Source: CAD feature listing. Evaluate the final solid. Frame: model axes, mm. Round coordinates to 2 decimals unless told otherwise and drop trailing zeros. Order: outer loops, then holes, each group sorted by start corner. A loop starts at its lowest first (then second) coordinate and runs counter-clockwise, first axis right, second up. Notation, with made-up numbers: M 38.5,58.25 L 83.5,58.25 A32 cw 83.5,84.25 Z; hole C 31.5,-5.5 d1. An arc over 180 degrees is marked long. Answer as CSV lines item,"result". Start each with the question number.
Item 1: Line query: line 1 (X direction, y = 1, z = 0); line 2 (X direction, y = 0.25, z = -11.43); line 3 (X direction, y = 4.75, z = 1). Output: solid intervals per line, ascending. Write a range as [from, to].
Item 2: Pull-direction query (Z, two-part tool) for faces 1 (the face through (-47, 5.08, 0)), 2 (the face through (-45.05, 0.07, 12.29)), 3 (the face through (-122.64, 0.03, -1.07)), 4 (the face through (-88.502, 0.763, 2.423)); classes: +Z half, -Z half, draft (parallel to the pull), parting line (faces both ways), or undercut.
Item 3: Section query C-C on y = -3.5. Return the cut outline in (x, z).
Item 4: Section query D-D on x = -94. Return the cut outline in (y, z), plus the area to 3 significant figures.
Item 5: Section query A-A on y = 0. Return the cut outline in (x, z).
Item 6: Section query B-B on z = 0. Return the cut outline in (x, y).
Item 7: First-contact query: P1, Ø3.5, axis at x = -47.13, z = -11.43, coming from the +Y side; P2, Ø3, axis at x = -55, z = 2, coming from the -Y side; P3, Ø1, axis at x = -116, y = -2, coming from the -Z side; P4, Ø6, axis at y = -3.5, z = -11.5, coming from the -X side. Flat tips, straight axial feed; report the tip coordinate or a pass-through.
from build123d import *

# Parameters (mm, degrees)
BOSS_EXTRUDE1_DEPTH = 5.08
CUT_EXTRUDE1_REACH  = 12.16
SKETCH4_R           = 2.2479
SKETCH5_R           = 2.54
BOSS_EXTRUDE2_DEPTH = 76.2
CUT_EXTRUDE5_REACH  = 9.62
SKETCH6_R           = 1.27


with BuildPart() as part:
    # Sketch2 → Boss-Extrude1 (new body, symmetric)
    with BuildSketch(Plane(origin=(0, 0, 0), x_dir=(1, 0, 0), z_dir=(0, 1, 0))):
        with BuildLine():
            Line((-50.935337995, 2.421627074), (-50.935337995, -2.138056527))
            Line((-50.935337995, -2.138056527), (-50.935337995, -11.43))
            ThreePointArc((-50.935337995, -11.43), (-47.125337995, -15.24), (-43.315337995, -11.43))
            Line((-43.315337995, -11.43), (-43.315337995, 11.43))
            ThreePointArc((-43.315337995, 11.43), (-47.125337995, 15.24), (-50.935337995, 11.43))
            Line((-50.935337995, 11.43), (-50.935337995, 2.421627074))
        make_face()
    extrude(amount=BOSS_EXTRUDE1_DEPTH, both=True)

    # Sketch4 → Cut-Extrude1 (cut, up to next)
    with BuildSketch(Plane(origin=(0, 5.08, 0), x_dir=(1, 0, 0), z_dir=(0, 1, 0)), mode=Mode.PRIVATE) as cut_extrude1_sk1:
        with Locations((-47.125337995, 11.43)):
            Circle(SKETCH4_R)
    cut_extrude1_tool1 = extrude(cut_extrude1_sk1.sketch, amount=-CUT_EXTRUDE1_REACH, mode=Mode.PRIVATE) & part.part
    add(cut_extrude1_tool1.solids().sort_by_distance((-47.125338, 5.08, -11.43))[0], mode=Mode.SUBTRACT)
    # Sketch4 → Cut-Extrude1 (cut, up to next)
    with BuildSketch(Plane(origin=(0, 5.08, 0), x_dir=(1, 0, 0), z_dir=(0, 1, 0)), mode=Mode.PRIVATE) as cut_extrude1_sk2:
        with Locations((-47.125337995, -11.43)):
            Circle(SKETCH4_R)
    cut_extrude1_tool2 = extrude(cut_extrude1_sk2.sketch, amount=-CUT_EXTRUDE1_REACH, mode=Mode.PRIVATE) & part.part
    add(cut_extrude1_tool2.solids().sort_by_distance((-47.125338, 5.08, 11.43))[0], mode=Mode.SUBTRACT)

    # Sketch5 → Boss-Extrude2 (add)
    with BuildSketch(Plane.ZY.offset(50.935337995)):
        Circle(SKETCH5_R)
    extrude(amount=BOSS_EXTRUDE2_DEPTH)

    # Sketch6 → Cut-Extrude5 (cut, up to next)
    with BuildSketch(Plane(origin=(0, 2.54, 0), x_dir=(1, 0, 0), z_dir=(0, 1, 0)), mode=Mode.PRIVATE) as cut_extrude5_sk1:
        with Locations((-123.325337995, 0)):
            Circle(SKETCH6_R)
    cut_extrude5_tool1 = extrude(cut_extrude5_sk1.sketch, amount=-CUT_EXTRUDE5_REACH, mode=Mode.PRIVATE) & part.part
    add(cut_extrude5_tool1.solids().sort_by_distance((-123.325338, 2.54, 0))[0], mode=Mode.SUBTRACT)


solid = part.part
Results:
1,line 1,"[-127.14, -124.6], [-122.06, -43.32]"
1,line 2,"[-50.94, -49.37], [-44.88, -43.32]"
1,line 3,"[-50.94, -43.32]"
2,face 1,"draft"
2,face 2,"undercut"
2,face 3,"undercut"
2,face 4,"parting line"
3,outline,"M -50.94,-11.43 A3.81 ccw -43.32,-11.43 L -43.32,11.43 A3.81 ccw -50.94,11.43 Z; hole C -47.13,-11.43 d4.5; hole C -47.13,11.43 d4.5"
4,outline,"C 0,0 d5.08"
4,area,"20.3 mm^2"
5,outline,"M -127.14,-2.54 L -50.94,-2.54 L -50.94,-11.43 A3.81 ccw -43.32,-11.43 L -43.32,11.43 A3.81 ccw -50.94,11.43 L -50.94,2.54 L -127.14,2.54 Z; hole C -123.33,0 d2.54; hole C -47.13,-11.43 d4.5; hole C -47.13,11.43 d4.5"
6,outline,"M -127.14,-2.54 L -124.6,-2.54 L -124.6,2.54 L -127.14,2.54 Z; M -122.06,-2.54 L -50.94,-2.54 L -50.94,-5.08 L -43.32,-5.08 L -43.32,5.08 L -50.94,5.08 L -50.94,2.54 L -122.06,2.54 Z"
7,P1,"through"
7,P2,"y = -2.49"
7,P3,"z = -2.05"
7,P4,"x = -50.94"
